from build123d import *

# Parameters (mm, degrees)
BOSS_EXTRUDE1_DEPTH = 2
SKETCH7_W           = 5
SKETCH7_H           = 1.5
CUT_EXTRUDE1_DEPTH  = 1
SKETCH8_R           = 1
CUT_EXTRUDE2_DEPTH  = 5


with BuildPart() as part:
    # Sketch6 → Boss-Extrude1 (new body)
    with BuildSketch(Plane(origin=(0, -10, 0), x_dir=(1, 0, 0), z_dir=(0, 1, 0))):
        with BuildLine():
            Line((-46, -7), (-46, -43.5))
            ThreePointArc((-46, -43.5), (-45.267766953, -45.267766953), (-43.5, -46))
            Line((-43.5, -46), (43.5, -46))
            ThreePointArc((43.5, -46), (45.267766953, -45.267766953), (46, -43.5))
            Line((46, -43.5), (46, -7))
            Line((46, -7), (41, -7))
            Line((41, -7), (41, 7))
            Line((41, 7), (46, 7))
            Line((46, 7), (46, 43.5))
            ThreePointArc((46, 43.5), (45.267766953, 45.267766953), (43.5, 46))
            Line((43.5, 46), (-43.5, 46))
            ThreePointArc((-43.5, 46), (-45.267766953, 45.267766953), (-46, 43.5))
            Line((-46, 43.5), (-46, 7))
            Line((-46, 7), (-41, 7))
            Line((-41, 7), (-41, -7))
            Line((-41, -7), (-46, -7))
        make_face()
    extrude(amount=BOSS_EXTRUDE1_DEPTH)

    # Sketch7 → Cut-Extrude1 (cut)
    with BuildSketch(Plane(origin=(0, -8, 0), x_dir=(1, 0, 0), z_dir=(0, 1, 0))):
        with Locations((-43.5, 7.75)):
            Rectangle(SKETCH7_W, SKETCH7_H)
        with Locations((-43.5, -7.75)):
            Rectangle(SKETCH7_W, SKETCH7_H)
        with Locations((43.5, -7.75)):
            Rectangle(SKETCH7_W, SKETCH7_H)
        with Locations((43.5, 7.75)):
            Rectangle(SKETCH7_W, SKETCH7_H)
    extrude(amount=-CUT_EXTRUDE1_DEPTH, mode=Mode.SUBTRACT)

    # Sketch8 → Cut-Extrude2 (cut)
    with BuildSketch(Plane(origin=(0, -8, 0), x_dir=(1, 0, 0), z_dir=(0, 1, 0))):
        with Locations(Location((-43.5, 43.5, 0), (0, 0, 270))):
            Circle(SKETCH8_R)
        with Locations(Location((43.5, 43.5, 0), (0, 0, 270))):
            Circle(SKETCH8_R)
        with Locations(Location((-43.5, -43.5, 0), (0, 0, 270))):
            Circle(SKETCH8_R)
        with Locations(Location((43.5, -43.5, 0), (0, 0, 270))):
            Circle(SKETCH8_R)
        with Locations(Location((-28.5, 28.5, 0), (0, 0, 270))):
            Circle(SKETCH8_R)
        with Locations(Location((28.5, 28.5, 0), (0, 0, 270))):
            Circle(SKETCH8_R)
        with Locations(Location((-28.5, -28.5, 0), (0, 0, 270))):
            Circle(SKETCH8_R)
        with Locations(Location((28.5, -28.5, 0), (0, 0, 270))):
            Circle(SKETCH8_R)
    extrude(amount=-CUT_EXTRUDE2_DEPTH, mode=Mode.SUBTRACT)


solid = part.part
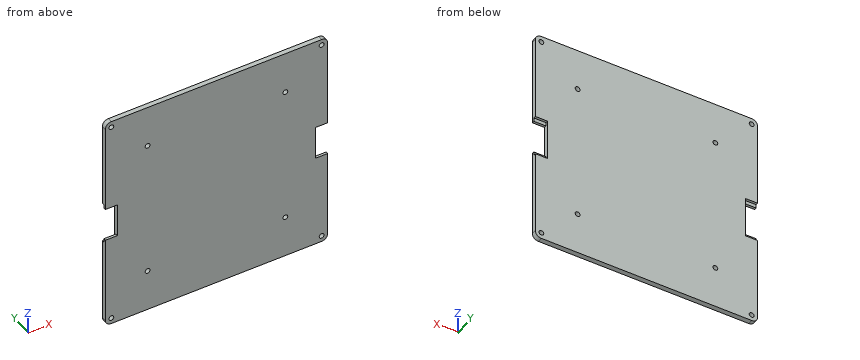
Input: part model. Units: mm. Frame: model coordinates. Coordinates: 2 decimals unless noted, no trailing zeros. Order: outer loops, then holes, each group sorted by start corner. A loop starts at its lowest first (then second) coordinate and runs counter-clockwise, first axis right, second up. Notation, with made-up numbers: M -9.75,-18.75 L 25.25,-18.75 A25 cw 25.25,5.25 Z; hole C -31,19 d4. An arc over 180 degrees is marked long. Answer as CSV lines item,"result".
1. First-contact query: P1, Ø1.6, axis at x = -28.5, z = -28.5, coming from the -Y side; P2, Ø1.2, axis at x = -44.5, z = -8, coming from the +Y side; P3, Ø1, axis at y = -9, z = -5.5, coming from the -X side; P4, Ø0.8, axis at x = -42.5, z = 7.5, coming from the +Y side. Flat tips, straight axial feed; report the tip coordinate or a pass-through.
Reported:
P1,"through"
P2,"y = -8"
P3,"x = -41"
P4,"y = -9"
2. Material intervals for line 1 (X direction, y = -9.1, z = 28.5); line 2 (X direction, y = -8.2, z = -7.5), sorted ascending. Write a range as from..to.
Reported:
line 1,"-46..-29.5, -27.5..27.5, 29.5..46"
line 2,"-41..41"
3. Section A-A (z = 5.5). Return the cut outline in (x, y), then the cut area to 3 significant figures.
Reported:
outline,"M -41,-10 L 41,-10 L 41,-8 L -41,-8 Z"
area,"164 mm2"
